from build123d import *

# Parameters (mm, degrees)
F0_R     = 19.626039
F1_DEPTH = 2.5
F2_R     = 2
F3_R     = 15


with BuildPart() as f1:
    # F0 (on Top) → F1 (new body, symmetric)
    with BuildSketch(Plane.XY):
        with BuildLine():
            Line((370, 300), (250, 300))
            Line((250, 300), (250, 0))
            Line((250, 0), (270, 0))
            ThreePointArc((270, 0), (295.658351, 158.113883), (370, 300))
        make_face()
        with Locations((294.626039, 255.373961)):
            Circle(F0_R, mode=Mode.SUBTRACT)
        with Locations((294.626039, 255.373961)):
            Circle(F0_R)
    extrude(amount=F1_DEPTH, both=True)

    # F2
    f2_edges = [f1.edges().sort_by_distance(p)[0] for p in [
        (250, 0, 0),
        (370, 300, 0),
    ]]
    fillet(f2_edges, radius=F2_R)

    # F3
    f3_edges = [f1.edges().sort_by_distance(p)[0] for p in [
        (270, 0, 0),
    ]]
    fillet(f3_edges, radius=F3_R)


solid = f1.part
Here's how the part is built. I have some questions about the finished solid (model axes, mm). Coordinates: 2 decimals unless noted, no trailing zeros. Loops run counter-clockwise (first coordinate to the right, second up) from the corner with the lowest first, then second, coordinate; pieces in that order, holes last.
1. Imagine slicing it at B-B, the plane x = 339. Please give me the cut outline in (y, z), and give its area (3 significant figures).
2. I need wall thicknesses on L1, parallel to X at y = 273.5, z = -0.5; L2, parallel to Y at x = 313.5, z = 1.55; L3, parallel to X at y = 285.5, z = 2. Which ranges of each line are inside material? Lowest first, please.
3. Imagine slicing it at A-A, the plane z = -0.75. Please give me the cut outline in (x, y), and give its area (3 significant figures).
4. Imagine slicing it at C-C, the plane y = 45.5. Please give me the cut outline in (x, z).
Taken from the geometry:
1. outline: (253.45, -2.5) - (300, -2.5) - (300, 2.5) - (253.45, 2.5) - close
1. area: 233 mm2
2. L1: x = 250 to 351.43
2. L2: y = 203.98 to 300
2. L3: x = 250 to 359.52
3. outline: (250, 2) arc R2 ccw to (252, 0) - (255.22, 0) arc R15 ccw to (270.21, 14.56) arc R500 cw to (367.63, 296.81) arc R2 ccw to (366.02, 300) - (250, 300) - close
3. area: 15,500 mm2
4. outline: (250, -2.5) - (272.07, -2.5) - (272.07, 2.5) - (250, 2.5) - close
